Source: three-view drawing plus pictorial views. Frame: mm from the lowest corner of the part. Round coordinates to 2 decimals unless told otherwise and drop trailing zeros. Order: outer loops, then holes, each group sorted by start corner. A loop starts at its lowest first (then second) coordinate and runs counter-clockwise, first axis right, second up. Notation, with made-up numbers: (20, 23.5) -> (51, 23.5) arc R30 ccw to (51, 59.5) -> close; hole circle Ø8 at (65.25, 42). An arc over 180 degrees is marked (long way). Use a Markdown table: item, result.
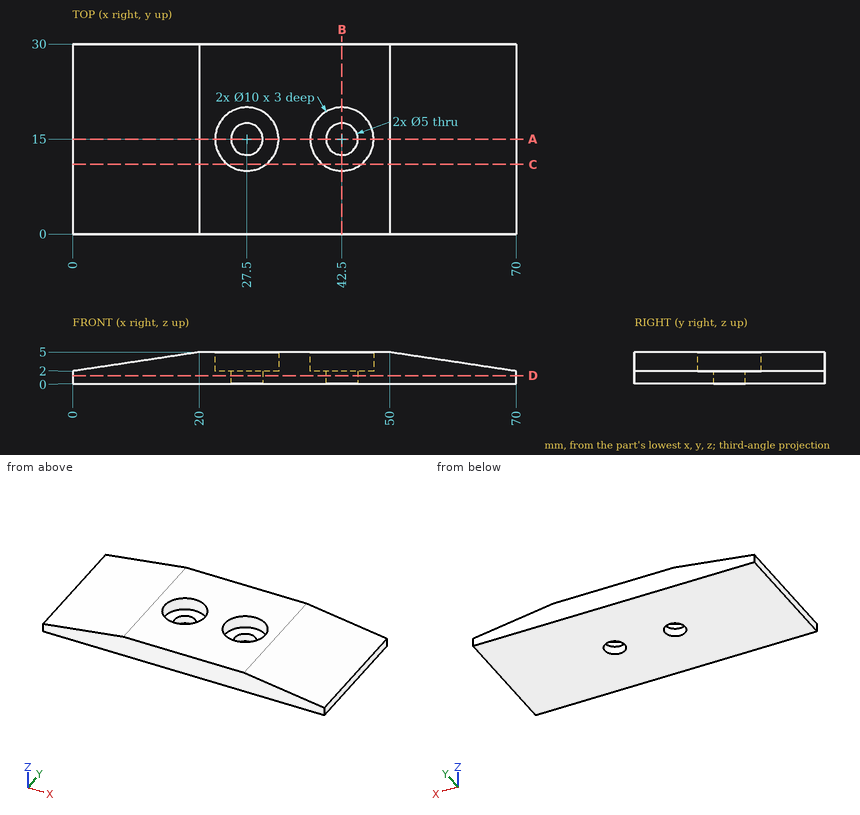
1) Cut plane C-C on y = 11. Return loops of the section in (x, z), and give its area (3 significant figures).
Results found:
| item | result |
|---|---|
| outline | (0, 0) -> (70, 0) -> (70, 2) -> (50, 5) -> (45.5, 5) -> (45.5, 2) -> (39.5, 2) -> (39.5, 5) -> (30.5, 5) -> (30.5, 2) -> (24.5, 2) -> (24.5, 5) -> (20, 5) -> (0, 2) -> close |
| area | 254 mm² |
2) Pin query (flat end, axial travel): pin 1 Ø1 at (x, z) = (59, 2) entering from -Y; pin 2 Ø3 at (x, y) = (43, 14) entering from +Z. Return the tip coordinate at first contact, or that it passes through.
Results found:
| item | result |
|---|---|
| pin 1 | stops at y = 0 |
| pin 2 | stops at z = 2 |
3) Cut plane B-B on x = 42.5. Return loops of the section in (y, z).
Results found:
| item | result |
|---|---|
| outline | (0, 0) -> (12.5, 0) -> (12.5, 2) -> (10, 2) -> (10, 5) -> (0, 5) -> close; (17.5, 0) -> (30, 0) -> (30, 5) -> (20, 5) -> (20, 2) -> (17.5, 2) -> close |
4) Line query: L1, parallel to Y at x = 27.5, z = 2.6; L2, parallel to Y at x = 42.5, z = 0.55; L3, parallel to Z at x = 28, y = 10.5. Output: solid intervals per line, ascending. Write a range as [from, to].
Results found:
| item | result |
|---|---|
| L1 | y = [0, 10], [20, 30] |
| L2 | y = [0, 12.5], [17.5, 30] |
| L3 | z = [0, 2] |
5) Cut plane D-D on z = 1.3. Return loops of the section in (x, y).
Results found:
| item | result |
|---|---|
| outline | (0, 0) -> (70, 0) -> (70, 30) -> (0, 30) -> close; hole circle Ø5 at (27.5, 15); hole circle Ø5 at (42.5, 15) |
6) Cut plane A-A on y = 15. Return loops of the section in (x, z).
Results found:
| item | result |
|---|---|
| outline | (0, 0) -> (25, 0) -> (25, 2) -> (22.5, 2) -> (22.5, 5) -> (20, 5) -> (0, 2) -> close; (30, 0) -> (40, 0) -> (40, 2) -> (37.5, 2) -> (37.5, 5) -> (32.5, 5) -> (32.5, 2) -> (30, 2) -> close; (45, 0) -> (70, 0) -> (70, 2) -> (50, 5) -> (47.5, 5) -> (47.5, 2) -> (45, 2) -> close |
